from build123d import *

# Parameters (mm, degrees)
SKETCH18_R          = 1.905
SKETCH18_R_2        = 3.175
SKETCH18_R_3        = 6.35
SKETCH18_R_4        = 2.5
SKETCH18_R_5        = 10.922
BOSS_EXTRUDE4_DEPTH = 6.35
CHAMFER1_SIZE       = 2.54
SKETCH19_R          = 32.808821981
BOSS_EXTRUDE5_DEPTH = 6.35
SKETCH20_R          = 6.0325
CUT_EXTRUDE1_DEPTH  = 6.35
SKETCH22_W          = 20
SKETCH22_H          = 6.35
BOSS_EXTRUDE6_DEPTH = 20.32
FILLET1_R           = 2.54


with BuildPart() as part:
    # Sketch18 → Boss-Extrude4 (new body)
    with BuildSketch(Plane.XY):
        with BuildLine():
            Line((0, 0), (-265.604745697, 0))
            ThreePointArc((-265.604745697, 0), (-298.882523776, 76.131915965), (-307.699061234, 158.75))
            Line((-307.699061234, 158.75), (-307.699061234, 165.1))
            ThreePointArc((-307.699061234, 165.1), (-305.839189294, 169.590128061), (-301.349061234, 171.45))
            Line((-301.349061234, 171.45), (-231.499061234, 171.45))
            Line((-231.499061234, 171.45), (-159.473782125, 158.75))
            Line((-159.473782125, 158.75), (-28.014368889, 158.75))
            ThreePointArc((-28.014368889, 158.75), (-23.851207857, 157.194850386), (-21.727208485, 153.291130779))
            Line((-21.727208485, 153.291130779), (0, 0))
        make_face()
        with Locations((-180.594, 136.144)):
            Circle(SKETCH18_R, mode=Mode.SUBTRACT)
        with Locations((-11.423473622, 24.034728138)):
            Circle(SKETCH18_R_2, mode=Mode.SUBTRACT)
        with Locations((-27.253356194, 124.406511892)):
            Circle(SKETCH18_R_2, mode=Mode.SUBTRACT)
        with Locations((-35.200938766, 146.05)):
            Circle(SKETCH18_R_3, mode=Mode.SUBTRACT)
        with Locations((-301.900938766, 146.05)):
            Circle(SKETCH18_R_2, mode=Mode.SUBTRACT)
        with Locations((-301.569673588, 132.761391752)):
            Circle(SKETCH18_R_2, mode=Mode.SUBTRACT)
        with Locations((-300.579872803, 119.537524267)):
            Circle(SKETCH18_R_2, mode=Mode.SUBTRACT)
        with Locations((-298.943543444, 106.442822899)):
            Circle(SKETCH18_R_2, mode=Mode.SUBTRACT)
        with Locations((-239.568937637, 24.034728138)):
            Circle(SKETCH18_R_2, mode=Mode.SUBTRACT)
        with Locations((-286.962142025, 164.850708953)):
            Circle(SKETCH18_R_2, mode=Mode.SUBTRACT)
        with Locations((-187.097045256, 107.95)):
            Circle(SKETCH18_R_4, mode=Mode.SUBTRACT)
        with Locations((-180.594, 105.156)):
            Circle(SKETCH18_R, mode=Mode.SUBTRACT)
        with Locations((-165.1, 120.65)):
            Circle(SKETCH18_R_5, mode=Mode.SUBTRACT)
        with Locations((-165.1, 146.05)):
            Circle(SKETCH18_R_4, mode=Mode.SUBTRACT)
        with Locations((-149.606, 105.156)):
            Circle(SKETCH18_R, mode=Mode.SUBTRACT)
        with Locations((-149.606, 136.144)):
            Circle(SKETCH18_R, mode=Mode.SUBTRACT)
        with Locations((-143.102954744, 107.95)):
            Circle(SKETCH18_R_4, mode=Mode.SUBTRACT)
    extrude(amount=BOSS_EXTRUDE4_DEPTH)

    # Chamfer1
    chamfer1_edges = [part.edges().sort_by_distance(p)[0] for p in [
        (-14.598473622, 24.034728138, 0),
        (-30.428356194, 124.406511892, 0),
        (-242.743937637, 24.034728138, 0),
        (-290.137142025, 164.850708953, 0),
    ]]
    chamfer(chamfer1_edges, length=CHAMFER1_SIZE)

    # Sketch19 → Boss-Extrude5 (add)
    with BuildSketch(Plane(origin=(0, 0, 0), x_dir=(-1, 0, 0), z_dir=(0, 0, -1))):
        with Locations((165.1, 120.65)):
            Circle(SKETCH19_R)
    extrude(amount=-BOSS_EXTRUDE5_DEPTH)

    # Sketch20 → Cut-Extrude1 (cut)
    with BuildSketch(Plane(origin=(0, 0, 0), x_dir=(-1, 0, 0), z_dir=(0, 0, -1))):
        with Locations((112.843509564, 96.674296134)):
            Circle(SKETCH20_R)
    extrude(amount=-CUT_EXTRUDE1_DEPTH, mode=Mode.SUBTRACT)

    # Sketch22 → Boss-Extrude6 (add)
    with BuildSketch(Plane.XZ):
        with Locations((-57.384832148, 3.175)):
            Rectangle(SKETCH22_W, SKETCH22_H)
        with Locations((-255.604745697, 3.175)):
            Rectangle(SKETCH22_W, SKETCH22_H)
    extrude(amount=BOSS_EXTRUDE6_DEPTH)

    # Fillet1
    fillet1_edges = [part.edges().sort_by_distance(p)[0] for p in [
        (-67.384832148, -20.32, 3.175),
        (-47.384832148, -20.32, 3.175),
        (-265.604745697, -20.32, 3.175),
        (-245.604745697, -20.32, 3.175),
    ]]
    fillet(fillet1_edges, radius=FILLET1_R)


solid = part.part
Build history of the part. All positions in model axes, mm. A direction names the side the tool comes from. Give positions to 0.01 mm unless a question says otherwise; leave off trailing zeros. Loops run counter-clockwise (first coordinate to the right, second up) from the corner with the lowest first, then second, coordinate; pieces in that order, holes last. Notation, with made-up numbers: (76, 68) -> (106, 68) arc R13 ccw to (106, 90) -> close; hole circle Ø2 at (89.25, 37.5). An arc over 180 degrees is marked (long way). Answer in a Markdown table with one row per item.
Item 1: Flat gauge pins, fed straight in: P1, Ø2, axis at x = -168, z = 5, coming from the +Y side; P2, Ø3, axis at x = -81, z = 3, coming from the +Y side; P3, Ø3, axis at x = -163, z = 3.5, coming from the +Y side. Where does each tip first touch, or does it go through?
Findings below:
| item | result |
|---|---|
| P1 | stops at y = 160.43 |
| P2 | stops at y = 158.75 |
| P3 | stops at y = 159.64 |
Item 2: Probe line 1 along Y through (x, z) = (-64.5, 4); line 2 along Y through (x, z) = (-288, 1.25); line 3 along X through (y, z) = (97.5, 5). List the from-to ranges inside material, lowest first. Write a range as [from, to].
Findings below:
| item | result |
|---|---|
| line 1 | y = [-20.32, 158.75] |
| line 2 | y = [43.54, 160.51], [169.19, 171.45] |
| line 3 | x = [-303.64, -118.82], [-106.87, -13.82] |
Item 3: Tool access for faces 4 (the flat face through (-307.699, 162, 3)), 5 (the flat face through (-265.605, -9, 3)), 6 (the flat face through (-155, 0, 3)): list every direction of +Z, -Z, +X, -X, +Y, -Y with a clear straight run to the whole face (end or side of a thin tool).
Findings below:
| item | result |
|---|---|
| face 4 | +Z, -Z, -X, +Y |
| face 5 | +Z, -Z, -X, -Y |
| face 6 | +Z, -Z, -Y |
Item 4: Mould opens along Y. For faces 1 (the flat face through (-156, 77, 0)), 2 (the conical face through (-9.6, 26.8, 2.4)), 3 (the flat face through (-23, 0, 3)) say: pulls with the +Y half, pulls with the -Y half, needs draft (parallel to the pull), parting line crosses it, or undercut.
Findings below:
| item | result |
|---|---|
| face 1 | needs draft |
| face 2 | undercut |
| face 3 | pulls with the -Y half |
Item 5: Slice it at A-A on y = 146.05. Write the cut outline in (x, z).
Findings below:
| item | result |
|---|---|
| outline | (-307.99, 0) -> (-305.08, 0) -> (-305.08, 6.35) -> (-307.99, 6.35) -> close; (-298.73, 0) -> (-41.55, 0) -> (-41.55, 6.35) -> (-298.73, 6.35) -> close; (-28.85, 0) -> (-20.7, 0) -> (-20.7, 6.35) -> (-28.85, 6.35) -> close |
Item 6: Slice it at D-D on y = 54.5. Write the cut outline in (x, z).
Findings below:
| item | result |
|---|---|
| outline | (-292.17, 0) -> (-7.72, 0) -> (-7.72, 6.35) -> (-292.17, 6.35) -> close |
Item 7: Slice it at C-C on x = -135. Write the cut outline in (y, z), plus the area to 3 significant figures.
Findings below:
| item | result |
|---|---|
| outline | (0, 0) -> (158.75, 0) -> (158.75, 6.35) -> (0, 6.35) -> close |
| area | 1,010 mm² |
Item 8: Slice it at B-B on z = 3.5. Give the number of separate pieces and of enclosed holes in the cut face, plus the area to 3 significant figures.
Findings below:
| item | result |
|---|---|
| separate pieces | 1 |
| enclosed holes | 10 |
| area | 46,800 mm² |
